Part model, mm, in its own coordinate system. A direction names the side the tool comes from. Coordinates: 2 decimals unless noted, no trailing zeros. Order: outer loops, then holes, each group sorted by start corner. A loop starts at its lowest first (then second) coordinate and runs counter-clockwise, first axis right, second up. Notation, with made-up numbers: (87.5, 13.25) - (135.5, 13.25) arc R13 ccw to (135.5, 38.25) - close; hole circle Ø1 at (16, 85.25). An arc over 180 degrees is marked (long way). Use a Markdown table: item, result. Add a question column.
1) Wall check: L1, parallel to X at y = 4, z = -36; L2, parallel to X at y = 3.95, z = -40; L3, parallel to Z at x = -51, y = 3.35. Give the ranges that are in metal, low to high. Write a range as [from, to].
2) Saw through at B-B on z = -40. List the corners of the cut face in (x, y), then the cut area to 3 significant figures.
3) Tool access for faces 1 (the face through (73, 3, -49)), 2 (the face through (-20, 2, 1)): list every direction of +Z, -Z, +X, -X, +Y, -Y with a clear straight run to the whole face (end or side of a thin tool).
4) Saw through at C-C on x = -35. List the corners of the cut face in (y, z).
5) Saw through at D-D on x = -50. List the corners of the cut face in (y, z).
6) Saw through at A-A on z = -2. List the corners of the cut face in (x, y), then the cut area to 3 significant figures.
7) Drop flat-ended pins along their axis: P1, Ø5.5, axis at x = -35, z = -36, coming from the -Y side; P2, Ø3, axis at x = -50, z = -40, coming from the -Y side. Give the stop position or say it passes through.
8) Two-plate mould, pull along Z, no slides. Class faces 3 (the face through (-34, 0, -12)), 4 (the face through (-1, 2, 50)), 5 (the face through (70, 2, 1)): +Z half, -Z half, draft (parallel to the pull), parting line (faces both ways), or undercut.
```python
from build123d import *

# Parameters (mm, degrees)
SKETCH1_W           = 150
SKETCH1_H           = 100
SKETCH1_W_2         = 90
SKETCH1_H_2         = 90
BOSS_EXTRUDE1_DEPTH = 5
FILLET1_R           = 5
SKETCH2_R           = 3.5
SKETCH2_R_2         = 2.5
SKETCH2_R_3         = 1.75
SKETCH2_R_4         = 4
SKETCH2_W           = 20
SKETCH2_H           = 3
CUT_EXTRUDE3_DEPTH  = 5


with BuildPart() as part:
    # Sketch1 → Boss-Extrude1 (new body)
    with BuildSketch(Plane(origin=(0, 0, 0), x_dir=(1, 0, 0), z_dir=(0, 1, 0))):
        Rectangle(SKETCH1_W, SKETCH1_H)
        with Locations((25, 0)):
            Rectangle(SKETCH1_W_2, SKETCH1_H_2, mode=Mode.SUBTRACT)
    extrude(amount=BOSS_EXTRUDE1_DEPTH)

    # Fillet1
    fillet1_edges = [part.edges().sort_by_distance(p)[0] for p in [
        (75, 2.5, 50),
        (-75, 2.5, 50),
        (-75, 2.5, -50),
        (75, 2.5, -50),
    ]]
    fillet(fillet1_edges, radius=FILLET1_R)

    # Sketch2 → Cut-Extrude3 (cut)
    with BuildSketch(Plane(origin=(0, 5, 0), x_dir=(1, 0, 0), z_dir=(0, 1, 0))):
        with Locations(Location((-65, 40, 0), (0, 0, 270))):
            Circle(SKETCH2_R)
        with Locations(Location((-50, 40, 0), (0, 0, 270))):
            Circle(SKETCH2_R_2)
        with Locations((-35, 36)):
            Circle(SKETCH2_R_3)
        with Locations((-35, 40)):
            Circle(SKETCH2_R_4)
        with Locations((-47.5, -40)):
            Rectangle(SKETCH2_W, SKETCH2_H)
    extrude(amount=-CUT_EXTRUDE3_DEPTH, mode=Mode.SUBTRACT)


solid = part.part
```
Results are:
| question | item | result |
|---|---|---|
| 1 | L1 | [-75, -36.75], [-33.25, -20], [70, 75] |
| 1 | L2 | [-75, -68.5], [-61.5, -52.5], [-47.5, -39], [-31, -20], [70, 75] |
| 1 | L3 | [-50, -42.29], [-37.71, 38.5], [41.5, 50] |
| 2 | outline | (-75, 0) - (-68.5, 0) - (-68.5, 5) - (-75, 5) - close; (-61.5, 0) - (-52.5, 0) - (-52.5, 5) - (-61.5, 5) - close; (-47.5, 0) - (-39, 0) - (-39, 5) - (-47.5, 5) - close; (-31, 0) - (-20, 0) - (-20, 5) - (-31, 5) - close; (70, 0) - (75, 0) - (75, 5) - (70, 5) - close |
| 2 | area | 200 mm2 |
| 3 | face 1 | -Z, +X, +Y, -Y |
| 3 | face 2 | +Y, -Y |
| 4 | outline | (0, -50) - (5, -50) - (5, -44) - (0, -44) - close; (0, -34.25) - (5, -34.25) - (5, 50) - (0, 50) - close |
| 5 | outline | (0, -50) - (5, -50) - (5, -42.5) - (0, -42.5) - close; (0, -37.5) - (5, -37.5) - (5, 38.5) - (0, 38.5) - close; (0, 41.5) - (5, 41.5) - (5, 50) - (0, 50) - close |
| 6 | outline | (-75, 0) - (-20, 0) - (-20, 5) - (-75, 5) - close; (70, 0) - (75, 0) - (75, 5) - (70, 5) - close |
| 6 | area | 300 mm2 |
| 7 | P1 | y = 0 |
| 7 | P2 | through |
| 8 | face 3 | draft |
| 8 | face 4 | +Z half |
| 8 | face 5 | undercut |
